Read the model definition and answer for the solid it produces. Units are mm, in the model's axes. A direction names the side the tool comes from. Coordinates: 2 decimals unless noted, no trailing zeros. Loops run counter-clockwise (first coordinate to the right, second up) from the corner with the lowest first, then second, coordinate; pieces in that order, holes last.
from build123d import *

# Parameters (mm, degrees)
BOSS_EXTRUDE1_DEPTH     = 700
FILLET1_R               = 12
BOSS_EXTRUDE2_DEPTH     = 12
BOSS_EXTRUDE3_DEPTH     = 200
CUT_EXTRUDE1_DEPTH      = 785.28509614
CUT_EXTRUDE1_DEPTH_BACK = 785.28509614


with BuildPart() as part:
    # Sketch1 → Boss-Extrude1 (new body)
    with BuildSketch(Plane.XY):
        Polygon((-175, 0), (175, 0), (175, -59), (75, -59), (75, -100), (-75, -100), (-75, -59), (-175, -59), align=None)
    extrude(amount=BOSS_EXTRUDE1_DEPTH)

    # Fillet1
    fillet1_edges = [part.edges().sort_by_distance(p)[0] for p in [
        (-175, -29.5, 0),
        (175, -29.5, 700),
        (-175, -29.5, 700),
        (175, -29.5, 0),
    ]]
    fillet(fillet1_edges, radius=FILLET1_R)

    # Sketch2 → Boss-Extrude2 (add)
    with BuildSketch(Plane(origin=(0, 0, 0), x_dir=(1, 0, 0), z_dir=(0, 1, 0))):
        with BuildLine():
            Line((-62, -588), (-62, -438))
            ThreePointArc((-62, -438), (0, -376), (62, -438))
            Line((62, -438), (62, -588))
            ThreePointArc((62, -588), (0, -650), (-62, -588))
        make_face()
        with BuildLine():
            Line((-34.5, -588), (-34.5, -438))
            ThreePointArc((-34.5, -438), (0, -403.5), (34.5, -438))
            Line((34.5, -438), (34.5, -588))
            ThreePointArc((34.5, -588), (0, -622.5), (-34.5, -588))
        make_face(mode=Mode.SUBTRACT)
    extrude(amount=BOSS_EXTRUDE2_DEPTH)

    # Sketch4 → Boss-Extrude3 (add)
    with BuildSketch(Plane(origin=(125.406543764, 0, 295.439302816), x_dir=(-0.9205048534524398, 0, 0.39073112848927494), z_dir=(-0.39073112848927494, 0, -0.9205048534524398))):
        Polygon((-26.717356398, 0), (211.282643602, 0), (211.282643602, 312), (142.282643602, 312), (92.826407103, 225.085785562), (143.632232896, 225.404217347), (56.684794392, 72.60309761), (31.00611148, 116.443017514), (-26.717356398, 15), align=None)
    extrude(amount=BOSS_EXTRUDE3_DEPTH)

    # Sketch5 → Cut-Extrude1 (cut, two sides: drawn at the far end of the back side and taken through both)
    with BuildSketch(Plane(origin=(-194.486698886, 0, 82.554705765), x_dir=(0.39073112848927494, 0, 0.9205048534524398), z_dir=(-0.9205048534524398, 0, 0.39073112848927494)).offset(-CUT_EXTRUDE1_DEPTH_BACK)):
        with BuildLine():
            Line((208.953552507, 1623.592968805), (208.953552507, 312))
            ThreePointArc((208.953552507, 312), (220.953552507, 300), (232.953552507, 312))
            Line((232.953552507, 312), (232.953552507, 1623.592968805))
            Line((232.953552507, 1623.592968805), (232.953552507, 4246.778906414))
            Line((232.953552507, 4246.778906414), (208.953552507, 4246.778906414))
            Line((208.953552507, 4246.778906414), (208.953552507, 1623.592968805))
        make_face()
    extrude(amount=CUT_EXTRUDE1_DEPTH + CUT_EXTRUDE1_DEPTH_BACK, mode=Mode.SUBTRACT)


solid = part.part
Q1. Which of the six approach directions +Z, -Z, +X, -X, +Y, -Y give full straight-line access (tool end or side, diameter ignored) to faces 1 (the face through (0.76, 5.92, 622.49)), 2 (the face through (1.363, 5.916, 649.985)), 3 (the face through (-124, -59, 345))?
Findings below:
face 1: +Y
face 2: +Z, +Y
face 3: +Z, -Z, -X, -Y
Q2. Determine the mould class of faces 4 (the face through (1, -100, 345)), 5 (the face through (-1.363, 5.916, 376.015)), 6 (the face through (-21.648, 269.151, 250.745)) for opening direction Z: +Z half, -Z half, draft (parallel to the pull), parting line (faces both ways), or undercut.
Findings below:
face 4: draft
face 5: undercut
face 6: -Z half
Q3. Straight lines are drawn through the part: probe 1 along Y at (x, z) = (63.5, 618); probe 2 along Y at (x, z) = (150.5, 245.5); probe 3 along Y at (x, z) = (-82, 169). For each, find the intervals that lie inside material, in ascending order.
Findings below:
probe 1: y = -100 to 0
probe 2: y = -59 to 0
probe 3: y = -59 to 221.68, 225.39 to 310.65
Q4. A cutting plane is placed at C-C (x = -122.5). Give the vertices of the cut face in (y, z), then the cut area to 3 significant figures.
Findings below:
outline: (-59, 0) - (0, 0) - (0, 183.4) - (312, 183.4) - (312, 252.14) - (0, 252.14) - (0, 700) - (-59, 700) - close
area: 62,700 mm2
Q5. A cutting plane is placed at B-B (z = 85). Give the vertices of the cut face in (x, y).
Findings below:
outline: (-175, -59) - (-75, -59) - (-75, -100) - (75, -100) - (75, -59) - (175, -59) - (175, 0) - (-175, 0) - close
Q6. A cutting plane is placed at A-A (x = 9.5). Give the vertices of the cut face in (y, z), then the cut area to 3 significant figures.
Findings below:
outline: (-100, 0) - (0, 0) - (0, 127.37) - (99.34, 127.37) - (72.6, 167.45) - (194.27, 344.64) - (0, 344.64) - (0, 376.73) - (12, 376.73) - (12, 404.83) - (0, 404.83) - (0, 621.17) - (12, 621.17) - (12, 649.27) - (0, 649.27) - (0, 700) - (-100, 700) - close; (225.09, 259.95) - (283.24, 344.64) - (225.29, 344.64) - close
area: 100,000 mm2
Q7. Flat-ended cylindrical pins translate along their axes: pin 1 Ø1 at (x, y) = (-80, 126) entering from -Z; pin 2 Ø5 at (x, y) = (-120, 254.5) entering from +Z; pin 3 Ø13 at (y, z) = (8, 500) entering from -X. Find the tip coordinate at first contact, or state that the pin passes through.
Findings below:
pin 1: stops at z = 165.14
pin 2: stops at z = 263.92
pin 3: stops at x = -62
Q8. A cutting plane is placed at D-D (y = 191.5). Give the vertices of the cut face in (x, z).
Findings below:
outline: (-147.23, 193.89) - (-67.2, 159.92) - (10.95, 344.02) - (-69.08, 377.99) - close
